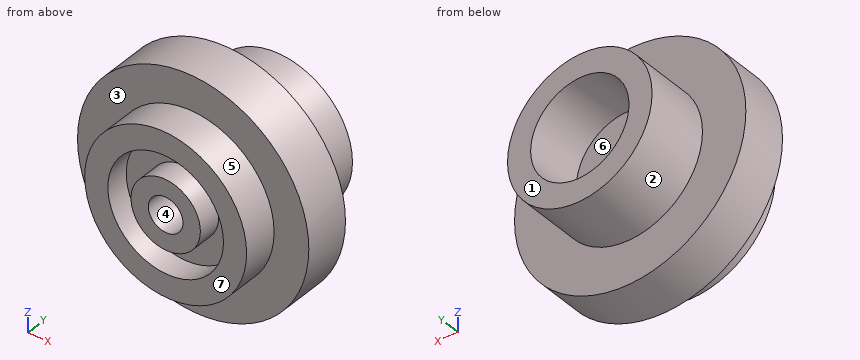
Autodesk Inventor part; units mm, degrees
ref_plane "YZ Plane" through (0, 0, 0) normal (1, 0, 0) x (0, 1, 0)
ref_plane "XZ Plane" through (0, 0, 0) normal (0, 1, 0) x (-1, 0, 0)
ref_plane "XY Plane" through (0, 0, 0) normal (0, 0, 1) x (1, 0, 0)
sketch "Эскиз1" plane through (0, 0, 0) normal (0, 0, 1) x (1, 0, 0)
  line L0 (6, 0) -> (12, 0)
  line L1 (12, 0) -> (12, 8)
  line L2 (12, 8) -> (20, 8)
  line L3 (20, 8) -> (20, 0)
  line L4 (20, 0) -> (28, 0)
  line L5 (28, 0) -> (28, 12)
  line L6 (28, 12) -> (40, 12)
  line L7 (40, 12) -> (40, 28)
  line L8 (40, 28) -> (25, 28)
  line L9 (25, 28) -> (25, 50)
  line L10 (25, 50) -> (17, 50)
  line L11 (17, 50) -> (17, 30)
  line L12 (17, 30) -> (6, 30)
  line L13 (6, 30) -> (6, 0)
  line L14 (6, 0) -> (0, 0)
  line L15 (0, 0) -> (0, 22.7372)
  dimension "d0" = 6
  dimension "d1" = 8
  dimension "d2" = 8
  dimension "d4" = 12
  dimension "d5" = 12
  dimension "d7" = 15
  dimension "d8" = 22
  dimension "d10" = 20
  dimension "d11" = 11
  dimension "d12" = 8
  dimension "d13" = 8
  dimension "d14" = 30
  dimension "d15" = 6
revolve "Вращение1" add sketch "Эскиз1" angle 360 about axis through (0, 0, 0) along (0, 1, 0)
properties part number "3"
Design review of the part built by this model. Coordinates are the model's own, in mm. Face numbers are marked on the shaded views. A direction names the side the tool comes from. Coordinates: 2 decimals unless noted, no trailing zeros. Loops run counter-clockwise (first coordinate to the right, second up) from the corner with the lowest first, then second, coordinate; pieces in that order, holes last.
Item 1: Wall thickness on L1, parallel to X at y = 7, z = 0; L2, parallel to X at y = 36, z = 0: over which ranges is each line inside the solid? List them lowest first.
Completed:
L1: x = -28 to -20, -12 to -6, 6 to 12, 20 to 28
L2: x = -25 to -17, 17 to 25
Item 2: For the marked faces 1, 2 and 3, list the 3-axis set-ups (+Z, -Z, +X, -X, +Y, -Y) from which the entire face can be reached by the end or side of a thin tool; tool diameter is ignored.
Completed:
face 1: +Z, -Z, +X, -X, +Y
face 2: +Y
face 3: -Y
Item 3: Add section D-D (x = 19). Write out the cut boundary in (y, z) (3 decimals), and give its area (3 significant figures).
Completed:
outline: (0, -20.567) - (12, -20.567) - (12, -35.199) - (28, -35.199) - (28, -16.248) - (50, -16.248) - (50, 16.248) - (28, 16.248) - (28, 35.199) - (12, 35.199) - (12, 20.567) - (0, 20.567) - (0, 6.245) - (8, 6.245) - (8, -6.245) - (0, -6.245) - close
area: 2,230 mm2
Item 4: Draft analysis for pull direction Z (two halves, no side actions). For the marked faces 4, 5, 6 and 7, state which applies: pulls with the +Z half, pulls with the -Z half, needs draft (parallel to the pull), parting line crosses it, or undercut.
Completed:
face 4: undercut
face 5: parting line crosses it
face 6: undercut
face 7: needs draft
Item 5: Add section A-A (x = 0). Write out the cut boundary in (y, z), and give its area (3 significant figures).
Completed:
outline: (0, -28) - (12, -28) - (12, -40) - (28, -40) - (28, -25) - (50, -25) - (50, -17) - (30, -17) - (30, -6) - (0, -6) - (0, -12) - (8, -12) - (8, -20) - (0, -20) - close; (0, 6) - (30, 6) - (30, 17) - (50, 17) - (50, 25) - (28, 25) - (28, 40) - (12, 40) - (12, 28) - (0, 28) - (0, 20) - (8, 20) - (8, 12) - (0, 12) - close
area: 1,880 mm2
Item 6: Add section B-B (z = 4). Write out the cut boundary in (x, y), and give its area (3 significant figures).
Completed:
outline: (-39.8, 12) - (-27.71, 12) - (-27.71, 0) - (-19.6, 0) - (-19.6, 8) - (-11.31, 8) - (-11.31, 0) - (-4.47, 0) - (-4.47, 30) - (-16.52, 30) - (-16.52, 50) - (-24.68, 50) - (-24.68, 28) - (-39.8, 28) - close; (4.47, 0) - (11.31, 0) - (11.31, 8) - (19.6, 8) - (19.6, 0) - (27.71, 0) - (27.71, 12) - (39.8, 12) - (39.8, 28) - (24.68, 28) - (24.68, 50) - (16.52, 50) - (16.52, 30) - (4.47, 30) - close
area: 1,960 mm2
Item 7: Add section C-C (y = 44.5). Write out the cut boundary in (x, z), and give its area (3 significant figures).
Completed:
outline: circle Ø50 at (0, 0); hole circle Ø34 at (0, 0)
area: 1,060 mm2
Item 8: Clearance check with flat-ended pins moving along their axes: pin 1 (1.5 mm diameter, centred on x = -32, z = -21, fed in from -Y); pin 2 (1.5 mm diameter, centred on x = 7.5, z = -13, fed in from +Y); pin 3 (12 mm diameter, centred on y = 10.5, z = -21.5, fed in from +X). State where each tip first meets the part, or that it passes through.
Completed:
pin 1: stops at y = 12
pin 2: stops at y = 30
pin 3: stops at x = 36.79
